```python
from build123d import *

# Parameters (mm, degrees)
SKETCH1_R           = 3.175
BOSS_EXTRUDE1_DEPTH = 17.1
BOSS_EXTRUDE2_DEPTH = 4.365625
BOSS_EXTRUDE3_DEPTH = 3.571875


with BuildPart() as part:
    # Sketch1 → Boss-Extrude1 (new body)
    with BuildSketch(Plane(origin=(0, 0, 0), x_dir=(1, 0, 0), z_dir=(0, 1, 0))):
        Circle(SKETCH1_R)
    extrude(amount=BOSS_EXTRUDE1_DEPTH)

    # Sketch2 → Boss-Extrude2 (add)
    with BuildSketch(Plane.XZ):
        Polygon((6.404947556, -0.373093671), (3.525582375, 5.360300458), (-2.879365181, 5.733394129), (-6.404947556, 0.373093671), (-3.525582375, -5.360300458), (2.879365181, -5.733394129), align=None)
    extrude(amount=BOSS_EXTRUDE2_DEPTH)

    # Sketch3 → Boss-Extrude3 (add)
    with BuildSketch(Plane(origin=(0, 17.1, 0), x_dir=(1, 0, 0), z_dir=(0, 1, 0))):
        Polygon((0, 6.415804866), (-5.55625, 3.207902433), (-5.55625, -3.207902433), (0, -6.415804866), (5.55625, -3.207902433), (5.55625, 3.207902433), align=None)
    extrude(amount=-BOSS_EXTRUDE3_DEPTH)


solid = part.part
```
Model file for the job. Use its own axes, mm. A direction names the side the tool comes from. Coordinates: 2 decimals unless noted, no trailing zeros. Loops run counter-clockwise (first coordinate to the right, second up) from the corner with the lowest first, then second, coordinate; pieces in that order, holes last. Notation, with made-up numbers: (47.5, 80) - (105.5, 80) arc R26 cw to (105.5, 116) - close; hole circle Ø4 at (5.5, -39). An arc over 180 degrees is marked (long way). Answer as a JSON object with one key per item and string values. Group by question number.
(1) Cut at D-D (z = 2.25). Give the cut face in (x, y).
(2) Probe line 1 along Y through (x, z) = (2.75, -4.25); line 2 along Y through (x, z) = (-2.75, -5); line 3 along X through (y, z) = (16, -0.75). List the from-to ranges inside material, lowest first.
(3) Cut at A-A (x = 4.25). Give the cut face in (y, z).
(4) Flat gauge pins, fed straight in: pin 1 (1.5 mm diameter, centred on y = 8.5, z = 4, fed in from -X); pin 2 (4 mm diameter, centred on y = 15.5, z = -0.5, fed in from -X); pin 3 (1 mm diameter, centred on x = -0.5, y = 1, fed in from +Z) (3 decimals); pin 4 (1.8 mm diameter, centred on y = 15, z = -1, fed in from +X). Where does each tip first touch, or does it go through?
(5) Two-plate mould, pull along Y, no slides. Class faces 5 (the face through (4.985, -2.152, 2.453)), 6 (the face through (0, -4.366, 0)), 7 (the face through (3, 0, 3)): released by +Y, released by -Y, zero draft, split by the parting line, or undercut.
(6) Tool access for faces 1 (the face through (-0.368, -2.152, -5.544)), 2 (the face through (0.368, -2.152, 5.544)), 3 (the face through (-2.8, 15.3, 4.8)), 4 (the face through (5.556, 15, 0)): list every direction of +Z, -Z, +X, -X, +Y, -Y with a clear straight run to the whole face (end or side of a thin tool).
(7) Cut at C-C (y = -0.5). Give the cut face in (x, z), then the cut area to 3 significant figures.
(8) Cut at B-B (z = -5). Give the cut face in (x, y), then the cut area to 3 significant figures.
Geometry says:
{
 "1": {"outline": "(-5.56, 13.53) - (-2.24, 13.53) - (-2.24, 0) - (-5.17, 0) - (-5.17, -4.37) - (5.09, -4.37) - (5.09, 0) - (2.24, 0) - (2.24, 13.53) - (5.56, 13.53) - (5.56, 17.1) - (-5.56, 17.1) - close"},
 "2": {"line 1": "y = -4.37 to 0, 13.53 to 17.1", "line 2": "y = -4.37 to 0", "line 3": "x = -5.56 to 5.56"},
 "3": {"outline": "(-4.37, -3.65) - (0, -3.65) - (0, 3.92) - (-4.37, 3.92) - close; (13.53, -3.96) - (17.1, -3.96) - (17.1, 3.96) - (13.53, 3.96) - close"},
 "4": {"pin 1": "passes through", "pin 2": "stops at x = -5.56", "pin 3": "stops at z = 3.175", "pin 4": "stops at x = 5.56"},
 "5": {"face 5": "zero draft", "face 6": "released by -Y", "face 7": "undercut"},
 "6": {"face 1": "-Z, -X, -Y", "face 2": "+Z, +X, -Y", "face 3": "+Z, -X, +Y", "face 4": "+Z, -Z, +X, +Y"},
 "7": {"outline": "(-6.4, 0.37) - (-3.53, -5.36) - (2.88, -5.73) - (6.4, -0.37) - (3.53, 5.36) - (-2.88, 5.73) - close", "area": "107 mm^2"},
 "8": {"outline": "(-3.71, -4.37) - (3.36, -4.37) - (3.36, 0) - (-3.71, 0) - close; (-2.45, 13.53) - (2.45, 13.53) - (2.45, 17.1) - (-2.45, 17.1) - close", "area": "48.4 mm^2"}
}
